```python
from build123d import *

# Parameters (mm, degrees)
SKETCH1_W           = 210
SKETCH1_H           = 250
BOSS_EXTRUDE1_DEPTH = 8
SKETCH_2_W          = 2.2
SKETCH_2_H          = 10.2
CUT_EXTRUDE_3_DEPTH = 164.444180074


with BuildPart() as part:
    # Sketch1 → Boss-Extrude1 (new body)
    with BuildSketch(Plane(origin=(0, 0, 0), x_dir=(1, 0, 0), z_dir=(0, 1, 0))):
        Rectangle(SKETCH1_W, SKETCH1_H)
    extrude(amount=BOSS_EXTRUDE1_DEPTH)

    # 草图2 → 切除-拉伸3 (cut, through all)
    with BuildSketch(Plane(origin=(0, 8, 0), x_dir=(1, 0, 0), z_dir=(0, 1, 0))):
        with Locations((0, -20)):
            Rectangle(SKETCH_2_W, SKETCH_2_H)
        Rectangle(SKETCH_2_W, SKETCH_2_H)
        with Locations((0, 20)):
            Rectangle(SKETCH_2_W, SKETCH_2_H)
        with Locations((0, 40)):
            Rectangle(SKETCH_2_W, SKETCH_2_H)
        with Locations((0, 60)):
            Rectangle(SKETCH_2_W, SKETCH_2_H)
        with Locations((0, 80)):
            Rectangle(SKETCH_2_W, SKETCH_2_H)
        with Locations((0, 100)):
            Rectangle(SKETCH_2_W, SKETCH_2_H)
        with Locations((0, -40)):
            Rectangle(SKETCH_2_W, SKETCH_2_H)
        with Locations((0, -60)):
            Rectangle(SKETCH_2_W, SKETCH_2_H)
        with Locations((0, -80)):
            Rectangle(SKETCH_2_W, SKETCH_2_H)
        with Locations((0, -100)):
            Rectangle(SKETCH_2_W, SKETCH_2_H)
        with Locations((98.9, 0)):
            Rectangle(SKETCH_2_W, SKETCH_2_H)
        with Locations((98.9, 20)):
            Rectangle(SKETCH_2_W, SKETCH_2_H)
        with Locations((-98.9, 0)):
            Rectangle(SKETCH_2_W, SKETCH_2_H)
        with Locations((98.9, 40)):
            Rectangle(SKETCH_2_W, SKETCH_2_H)
        with Locations((98.9, 60)):
            Rectangle(SKETCH_2_W, SKETCH_2_H)
        with Locations((98.9, 80)):
            Rectangle(SKETCH_2_W, SKETCH_2_H)
        with Locations((98.9, 100)):
            Rectangle(SKETCH_2_W, SKETCH_2_H)
        with Locations((98.9, -20)):
            Rectangle(SKETCH_2_W, SKETCH_2_H)
        with Locations((98.9, -40)):
            Rectangle(SKETCH_2_W, SKETCH_2_H)
        with Locations((98.9, -60)):
            Rectangle(SKETCH_2_W, SKETCH_2_H)
        with Locations((98.9, -80)):
            Rectangle(SKETCH_2_W, SKETCH_2_H)
        with Locations((98.9, -100)):
            Rectangle(SKETCH_2_W, SKETCH_2_H)
        with Locations((-98.9, 20)):
            Rectangle(SKETCH_2_W, SKETCH_2_H)
        with Locations((-98.9, 40)):
            Rectangle(SKETCH_2_W, SKETCH_2_H)
        with Locations((-98.9, 60)):
            Rectangle(SKETCH_2_W, SKETCH_2_H)
        with Locations((-98.9, 80)):
            Rectangle(SKETCH_2_W, SKETCH_2_H)
        with Locations((-98.9, 100)):
            Rectangle(SKETCH_2_W, SKETCH_2_H)
        with Locations((-98.9, -20)):
            Rectangle(SKETCH_2_W, SKETCH_2_H)
        with Locations((-98.9, -40)):
            Rectangle(SKETCH_2_W, SKETCH_2_H)
        with Locations((-98.9, -60)):
            Rectangle(SKETCH_2_W, SKETCH_2_H)
        with Locations((-98.9, -80)):
            Rectangle(SKETCH_2_W, SKETCH_2_H)
        with Locations((-98.9, -100)):
            Rectangle(SKETCH_2_W, SKETCH_2_H)
    extrude(amount=-CUT_EXTRUDE_3_DEPTH, mode=Mode.SUBTRACT)


solid = part.part
```
Design review of the part built by this model. Coordinates are the model's own, in mm. Give positions to 0.01 mm unless a question says otherwise; leave off trailing zeros. Order: outer loops, then holes, each group sorted by start corner. A loop starts at its lowest first (then second) coordinate and runs counter-clockwise, first axis right, second up. Notation, with made-up numbers: (61.25, 21.25) - (111.25, 21.25) arc R31 cw to (111.25, 55.25) - close; hole circle Ø3 at (-3, 41). An arc over 180 degrees is marked (long way). Use a Markdown table: item, result. Add a question column.
(1) Mouldability with a two-part tool opening along Z and no side actions: class faces 1 (the face through (-105, 4, 2)), 2 (the face through (100, 4, -40)) as +Z half, -Z half, draft (parallel to the pull), parting line (faces both ways), or undercut.
(2) Wall thickness on probe 1 along X at (y, z) = (5.5, -15): over which ranges is the line inside the solid? List them lowest first. Write a range as [from, to].
(3) Add section A-A on z = -80.5. Give the boundary of the cut face in (x, y), then the cut area to 3 significant figures.
Report:
| question | item | result |
|---|---|---|
| 1 | face 1 | draft |
| 1 | face 2 | undercut |
| 2 | probe 1 | x = [-105, -100], [-97.8, -1.1], [1.1, 97.8], [100, 105] |
| 3 | outline | (-105, 0) - (-100, 0) - (-100, 8) - (-105, 8) - close; (-97.8, 0) - (-1.1, 0) - (-1.1, 8) - (-97.8, 8) - close; (1.1, 0) - (97.8, 0) - (97.8, 8) - (1.1, 8) - close; (100, 0) - (105, 0) - (105, 8) - (100, 8) - close |
| 3 | area | 1,630 mm² |
